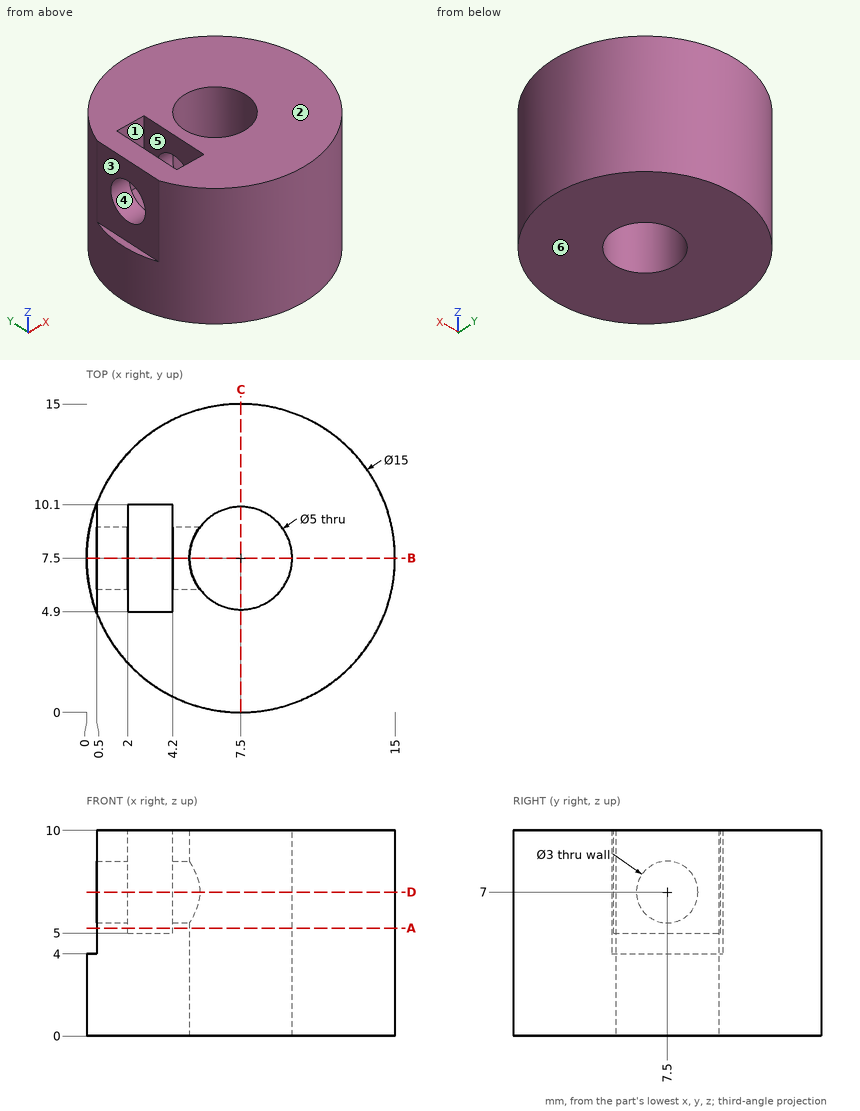
Input: dimensioned drawing with shaded views. Units: mm. Origin: part minimum x, y, z. A direction names the side the tool comes from. Give positions to 0.01 mm unless a question says otherwise; leave off trailing zeros. Loops run counter-clockwise (first coordinate to the right, second up) from the corner with the lowest first, then second, coordinate; pieces in that order, holes last. Notation, with made-up numbers: (31.5, -31) -> (55.5, -31) arc R9 ccw to (55.5, -17) -> close; hole circle Ø10 at (14.25, 13.25). An arc over 180 degrees is marked (long way). Return JSON: item names as keys, results as strings.
Item 1: Mould query, pull axis Z, two halves, no side actions, for the marked faces 4, 5 and 6. Classes: released by +Z, released by -Z, zero draft, split by the parting line, or undercut.
Filled in:
{"face 4": "undercut", "face 5": "zero draft", "face 6": "released by -Z"}
Item 2: Section D-D, the plane z = 7. Output: boundary loops of the cut face in (x, y), plus the area to 3 significant figures.
Filled in:
{"outline": "(0.5, 4.81) arc R7.5 ccw (long way) to (0.5, 10.19) -> (0.5, 9) -> (2, 9) -> (2, 10.1) -> (4.2, 10.1) -> (4.2, 9) -> (5.5, 9) arc R2.5 cw (long way) to (5.5, 6) -> (4.2, 6) -> (4.2, 4.9) -> (2, 4.9) -> (2, 6) -> (0.5, 6) -> close", "area": "136 mm^2"}
Item 3: Access query for the marked faces 1, 2 and 3. Directions: +Z, -Z, +X, -X, +Y, -Y. A direction counts if a zero-diameter tool reaches every point of the face in a straight line with its end or side. Return the directions, or none.
Filled in:
{"face 1": "+Z", "face 2": "+Z, +X, -X, +Y, -Y", "face 3": "+Z, -X, +Y, -Y"}
Item 4: Section C-C, the plane x = 7.5. Output: boundary loops of the cut face in (y, z), plus the area to 3 significant figures.
Filled in:
{"outline": "(0, 0) -> (5, 0) -> (5, 10) -> (0, 10) -> close; (10, 0) -> (15, 0) -> (15, 10) -> (10, 10) -> close", "area": "100 mm^2"}
Item 5: Line query: line 1 (Y direction, x = 7.5, z = 4.5); line 2 (X direction, y = 7.5, z = 4.25); line 3 (X direction, y = 9.5, z = 4.75). Output: solid intervals per line, ascending.
Filled in:
{"line 1": "0 to 5, 10 to 15", "line 2": "0.5 to 5, 10 to 15", "line 3": "0.5 to 6, 9 to 14.73"}
Item 6: Section B-B, the plane y = 7.5. Output: boundary loops of the cut face in (x, z).
Filled in:
{"outline": "(0, 0) -> (5, 0) -> (5, 5.5) -> (4.2, 5.5) -> (4.2, 5) -> (2, 5) -> (2, 5.5) -> (0.5, 5.5) -> (0.5, 4) -> (0, 4) -> close; (0.5, 8.5) -> (2, 8.5) -> (2, 10) -> (0.5, 10) -> close; (4.2, 8.5) -> (5, 8.5) -> (5, 10) -> (4.2, 10) -> close; (10, 0) -> (15, 0) -> (15, 10) -> (10, 10) -> close"}
Item 7: Pin query (flat end, axial travel): P1, Ø5, axis at y = 11.5, z = 2, coming from the -X side; P2, Ø6, axis at y = 8, z = 7.5, coming from the -X side; P3, Ø4, axis at x = 7.5, y = 7.5, coming from the +Z side; P4, Ø2.5, axis at y = 7.5, z = 7, coming from the -X side. Return the tip coordinate at first contact, or that it passes through.
Filled in:
{"P1": "x = 0.15", "P2": "x = 0.5", "P3": "through", "P4": "x = 9.67"}
Item 8: Section A-A, the plane z = 5.25. Output: boundary loops of the cut face in (x, y).
Filled in:
{"outline": "(0.5, 4.81) arc R7.5 ccw (long way) to (0.5, 10.19) -> close; hole (2, 4.9) -> (4.2, 4.9) -> (4.2, 10.1) -> (2, 10.1) -> close; hole circle Ø5 at (7.5, 7.5)"}
